The listing builds one solid part. Answer for the finished solid, in the listing's coordinates (mm). Coordinates: 2 decimals unless noted, no trailing zeros. Loops run counter-clockwise (first coordinate to the right, second up) from the corner with the lowest first, then second, coordinate; pieces in that order, holes last. Notation, with made-up numbers: (37.5, 69.25) - (81.5, 69.25) arc R24 ccw to (81.5, 82.25) - close; hole circle Ø3 at (-17.75, -0.5). An arc over 180 degrees is marked (long way). Write each question's results on one line, items separated by ' | '. Start each with the question number.
(1) Find section B-B on x = 499. Determine the outline of the cut face in (y, z), then the cut area to 3 significant figures.
(2) Given pin 1 Ø5 at (x, y) = (406.5, 205.5) entering from -Z; pin 2 Ø8 at (y, z) = (452, 14.5) entering from -X; pin 3 Ø6 at (x, z) = (-264.5, 25.5) entering from +Y; pin 4 Ø12 at (x, z) = (117.5, 22) entering from +Y, each flat-ended and moving along its own axis, determine where each tip first touches the part or whether it passes through.
(3) Find section C-C on z = 17.5. Determine the outline of the cut face in (x, y).
(4) Consider line 1 (Y direction, x = -311.5, z = 26); line 2 (Y direction, x = -224, z = 20.5); line 3 (X direction, y = -474, z = 8). Determine where each line is inside the solid, lowest interval first. Write a range as from..to.
(5) Find section A-A on y = -186. Determine the outline of the cut face in (x, z).
from build123d import *

# Parameters (mm, degrees)
F0_W     = 1700
F0_H     = 1300
F1_DEPTH = 30
F2_R     = 50


with BuildPart() as f1:
    # F0 (on Top) → F1 (new body)
    with BuildSketch(Plane.XY):
        Rectangle(F0_W, F0_H)
    extrude(amount=F1_DEPTH)

    # F2
    f2_edges = [f1.edges().sort_by_distance(p)[0] for p in [
        (-850, -650, 15),
        (-850, 650, 15),
        (850, -650, 15),
        (850, 650, 15),
    ]]
    fillet(f2_edges, radius=F2_R)

    # F6: sweep along a path in F5
    with BuildLine(Plane.XY.offset(30)) as f6_path:
        Line((800, 650), (-800, 650))
        ThreePointArc((-800, 650), (-835.3553390593, 635.3553390593), (-850, 600))
        Line((-850, 600), (-850, -600))
        ThreePointArc((-850, -600), (-835.3553390593, -635.3553390593), (-800, -650))
        Line((-800, -650), (800, -650))
        ThreePointArc((800, -650), (835.3553390593, -635.3553390593), (850, -600))
        Line((850, -600), (850, 600))
        ThreePointArc((850, 600), (835.3553390593, 635.3553390593), (800, 650))
    # F4 (on offset) → F6 (sweep)
    with BuildSketch(Plane.XZ.offset(600)):
        with BuildLine():
            Line((853.3333333333, 30), (850, 30))
            Line((850, 30), (850, 0))
            Line((850, 0), (900, 0))
            Line((900, 0), (865.3333333333, 26))
            ThreePointArc((865.3333333333, 26), (859.6578886537, 28.973665961), (853.3333333333, 30))
        make_face()
    sweep(path=f6_path.line)


solid = f1.part
Values:
1) outline: (-700, 0) - (700, 0) - (665.33, 26) arc R20 ccw to (653.33, 30) - (-653.33, 30) arc R20 ccw to (-665.33, 26) - close | area: 40,800 mm²
2) pin 1: stops at z = 0 | pin 2: stops at x = -886 | pin 3: stops at y = 670 | pin 4: stops at y = 678.67
3) outline: (-876.67, -600) arc R76.67 ccw to (-800, -676.67) - (800, -676.67) arc R76.67 ccw to (876.67, -600) - (876.67, 600) arc R76.67 ccw to (800, 676.67) - (-800, 676.67) arc R76.67 ccw to (-876.67, 600) - close
4) line 1: y = -665.33..665.33 | line 2: y = -672.67..672.67 | line 3: x = -889.33..889.33
5) outline: (-900, 0) - (900, 0) - (865.33, 26) arc R20 ccw to (853.33, 30) - (-853.33, 30) arc R20 ccw to (-865.33, 26) - close
